```python
from build123d import *

# Parameters (mm, degrees)
SKETCH2_R           = 1.1
BOSS_EXTRUDE1_DEPTH = 5
SKETCH3_OUTSIDE_W   = 130.75
SKETCH3_OUTSIDE_H   = 69.75
CUT_EXTRUDE1_DEPTH  = 3
CUT_EXTRUDE1_DRAFT  = -45
CUT_EXTRUDE2_DEPTH  = 3
CUT_EXTRUDE3_DEPTH  = 3
SKETCH6_R           = 3
CUT_EXTRUDE4_DEPTH  = 9
CUT_EXTRUDE5_DEPTH  = 3.5


with BuildPart() as part:
    # Sketch2 → Boss-Extrude1 (new body)
    with BuildSketch(Plane(origin=(0, 0, 0), x_dir=(1, 0, 0), z_dir=(0, 1, 0))):
        with BuildLine():
            Line((-36.162601626, 8.29200542), (-31.906454434, 8.29200542))
            Line((-31.906454434, 8.29200542), (32.553816284, 19.020616336))
            ThreePointArc((32.553816284, 19.020616336), (55.837398374, -0.70799458), (32.553816284, -20.436605496))
            Line((32.553816284, -20.436605496), (-31.906454434, -9.70799458))
            Line((-31.906454434, -9.70799458), (-36.162601626, -9.70799458))
            ThreePointArc((-36.162601626, -9.70799458), (-45.162601626, -0.70799458), (-36.162601626, 8.29200542))
        make_face()
        with Locations(Location((-42.162601626, -0.70799458, 0), (0, 0, 270))):
            Circle(SKETCH2_R, mode=Mode.SUBTRACT)
        with Locations(Location((54.337398374, -0.70799458, 0), (0, 0, 270))):
            Circle(SKETCH2_R, mode=Mode.SUBTRACT)
    extrude(amount=BOSS_EXTRUDE1_DEPTH)


with BuildPart() as cut_extrude1_tool:
    # Sketch3 outside → Cut-Extrude1 (with draft: the straight prism first)
    with BuildSketch(Plane(origin=(0, 5, 0), x_dir=(1, 0, 0), z_dir=(0, 1, 0))):
        with Locations((5.337, -0.708)):
            Rectangle(SKETCH3_OUTSIDE_W, SKETCH3_OUTSIDE_H)
        with BuildLine():
            ThreePointArc((-36.162601626, 5.29200542), (-42.162601626, -0.70799458), (-36.162601626, -6.70799458))
            Line((-36.162601626, -6.70799458), (-31.658503498, -6.70799458))
            Line((-31.658503498, -6.70799458), (33.046353598, -17.477313858))
            ThreePointArc((33.046353598, -17.477313858), (52.837398374, -0.70799458), (33.046353598, 16.061324698))
            Line((33.046353598, 16.061324698), (-31.658503498, 5.29200542))
            Line((-31.658503498, 5.29200542), (-36.162601626, 5.29200542))
        make_face(mode=Mode.SUBTRACT)
    extrude(amount=-CUT_EXTRUDE1_DEPTH)
    # Cut-Extrude1: the draft: its side faces are tilted about the plane it starts from
    cut_extrude1_sides = [cut_extrude1_tool.faces().sort_by_distance(p)[0] for p in [
        (5.337, 3.5, 35.583),
        (70.712, 3.5, 0.708),
        (5.337, 3.5, -34.167),
        (-60.038, 3.5, 0.708),
        (-33.910552562, 3.5, -5.29200542),
        (0.69392505, 3.5, -10.676665059),
        (52.837398374, 3.5, 0.70799458),
        (0.69392505, 3.5, 12.092654219),
        (-33.910552562, 3.5, 6.70799458),
        (-42.162601626, 3.5, 0.70799458),
    ]]
    draft(cut_extrude1_sides, Plane(origin=(0, 5, 0), x_dir=(1, 0, 0), z_dir=(0, 1, 0)), CUT_EXTRUDE1_DRAFT)


with BuildPart() as part_1:
    add(part.part)

    # Cut-Extrude1: cut by cut_extrude1_tool
    add(cut_extrude1_tool.part, mode=Mode.SUBTRACT)

    # Sketch4 → Cut-Extrude2 (cut)
    with BuildSketch(Plane(origin=(0, 5, 0), x_dir=(1, 0, 0), z_dir=(0, 1, 0))):
        with BuildLine():
            Line((-42.162601626, 1.29200542), (-47.036094896, 1.29200542))
            Line((-47.036094896, 1.29200542), (-47.036094896, -2.70799458))
            Line((-47.036094896, -2.70799458), (-42.162601626, -2.70799458))
            ThreePointArc((-42.162601626, -2.70799458), (-40.162601626, -0.70799458), (-42.162601626, 1.29200542))
        make_face()
    extrude(amount=-CUT_EXTRUDE2_DEPTH, mode=Mode.SUBTRACT)

    # Sketch5 → Cut-Extrude3 (cut)
    with BuildSketch(Plane(origin=(0, 5, 0), x_dir=(1, 0, 0), z_dir=(0, 1, 0))):
        with BuildLine():
            Line((54.337398374, 1.29200542), (57.452649993, 1.29200542))
            Line((57.452649993, 1.29200542), (57.452649993, -2.70799458))
            Line((57.452649993, -2.70799458), (54.337398374, -2.70799458))
            ThreePointArc((54.337398374, -2.70799458), (52.337398374, -0.70799458), (54.337398374, 1.29200542))
        make_face()
    extrude(amount=-CUT_EXTRUDE3_DEPTH, mode=Mode.SUBTRACT)

    # Sketch6 → Cut-Extrude4 (cut)
    with BuildSketch(Plane(origin=(0, 5, 0), x_dir=(1, 0, 0), z_dir=(0, 1, 0))):
        with Locations(Location((-32.662601626, -0.70799458, 0), (0, 0, 270))):
            Circle(SKETCH6_R)
    extrude(amount=-CUT_EXTRUDE4_DEPTH, mode=Mode.SUBTRACT)

    # Sketch7 → Cut-Extrude5 (cut)
    with BuildSketch(Plane.XZ):
        with BuildLine():
            Line((-37.079268293, 6.637557989), (33.240176152, 17.508424239))
            ThreePointArc((33.240176152, 17.508424239), (52.837398374, 0.70799458), (33.240176152, -16.092435079))
            Line((33.240176152, -16.092435079), (-37.079268293, -5.221568829))
            ThreePointArc((-37.079268293, -5.221568829), (-42.162601626, 0.70799458), (-37.079268293, 6.637557989))
        make_face()
    extrude(amount=-CUT_EXTRUDE5_DEPTH, mode=Mode.SUBTRACT)


solid = part_1.part
```
Source: CAD feature listing. Evaluate the final solid. Frame: model axes, mm. A direction names the side the tool comes from. Give positions to 0.01 mm unless a question says otherwise; leave off trailing zeros. Write each loop counter-clockwise with the first axis right and the second up, starting at its lowest first coordinate (ties: lowest second). Pieces come first, ordered by that corner, then holes. Notation, with made-up numbers: (-17, 55.25) - (16, 55.25) arc R18 cw to (16, 82.25) - close; hole circle Ø11 at (8, -18). An arc over 180 degrees is marked (long way). One line per item, written item: value. Start each with the question number.
Q1. Section query B-B, the plane x = -21. Return the cut outline in (y, z).
Q2. Set-up query: faces 4 (the face through (52.338, 3.854, 0.752)), 5 (the face through (-34, 1, 9.708)), 6 (the face through (-43, 3, 2.708)). Return all of +Z, -Z, +X, -X, +Y, -Y with unobstructed straight access to the full face (end or side cutting, diameter ignored); none if empty.
Q3. First-contact query: pin 1 Ø2 at (x, z) = (33.5, 5) entering from -Y; pin 2 Ø2 at (x, y) = (-44, 2.5) entering from -Z; pin 3 Ø3 at (x, y) = (-43.5, 4) entering from +Z. Flat tips, straight axial feed; report the tip coordinate or a pass-through.
Q4. Section query C-C, the plane x = 1.5. Return the cut outline in (y, z), then the cut area to 3 significant figures.
Q5. Draft query along Z for faces 1 (the face through (-34, 1, -8.292)), 2 (the face through (-1.427, 1.726, -10.733)), 3 (the face through (-40.671, 3.854, 6.252)). Return one class per face: +Z half, -Z half, draft (parallel to the pull), parting line (faces both ways), or undercut.
Q6. Material intervals for probe 1 along Y at (x, z) = (18, 10.5); probe 2 along X at (y, z) = (0.7, 5); probe 3 along Z at (x, y) = (29, 0.3), sorted ascending. Write a range as from..to.
Q7. Section query A-A, the plane y = 1.1. Return the cut outline in (x, z), then the cut area to 3 significant figures.
Answer:
1. outline: (0, -10.11) - (2, -10.11) - (5, -7.07) - (5, 8.48) - (2, 11.52) - (0, 11.52) - (0, 9.12) - (3.5, 9.12) - (3.5, -7.71) - (0, -7.71) - close
2. face 4: +X, +Y
2. face 5: +Z, -X, +Y, -Y
2. face 6: -X, +Y
3. pin 1: stops at y = 3.5
3. pin 2: stops at z = -4.98
3. pin 3: stops at z = 5.79
4. outline: (0, -13.85) - (2, -13.85) - (5, -10.81) - (5, 12.23) - (2, 15.27) - (0, 15.27) - (0, 12.6) - (3.5, 12.6) - (3.5, -11.19) - (0, -11.19) - close
4. area: 53.2 mm2
5. face 1: -Z half
5. face 2: undercut
5. face 3: +Z half
6. probe 1: y = 3.5..5
6. probe 2: x = -44.07..-40.36, 52.29..55.37
6. probe 3: z = -18.43..-15.44, 16.85..19.85
7. outline: (-36.16, -8.29) - (-31.91, -8.29) - (32.55, -19.02) arc R20 ccw (long way) to (32.55, 20.44) - (-31.91, 9.71) - (-36.16, 9.71) arc R9 ccw to start; hole (-42.06, -0.39) arc R6 ccw to (-37.08, -5.22) - (33.24, -16.09) arc R17 ccw (long way) to (33.24, 17.51) - (-37.08, 6.64) arc R6 ccw to (-42.06, 1.8) arc R1.1 ccw (long way) to start; hole circle Ø2.2 at (54.34, 0.71)
7. area: 623 mm2
